Read the model definition and answer for the solid it produces. Units are mm, in the model's axes. Give positions to 0.01 mm unless a question says otherwise; leave off trailing zeros. Order: outer loops, then holes, each group sorted by start corner. A loop starts at its lowest first (then second) coordinate and runs counter-clockwise, first axis right, second up. Notation, with made-up numbers: (23, 8) -> (58, 8) arc R17 ccw to (58, 39) -> close; hole circle Ø2 at (76.25, 24). An arc over 180 degrees is marked (long way). Answer as CSV lines item,"result". Start each with the question number.
1) Find section B-B (z = 2.5). Determine the outline of the cut face in (x, y).
2) Straight lines are drawn through the part: L1, parallel to X at y = 8, z = 3; L2, parallel to Y at x = -11.5, z = 5.5; L3, parallel to Z at x = 9, y = -3.5. For each, find the intervals that lie inside material, in ascending order. Write a range as from..to.
3) Find section A-A (y = 4). Determine the outline of the cut face in (x, z).
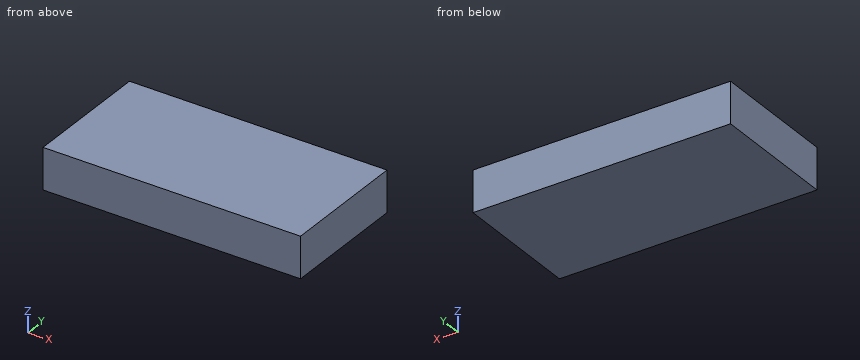
```python
from build123d import *

# Parameters (mm, degrees)
SKETCH_W     = 100
SKETCH_H     = 50
PAD_DEPTH    = 6
SKETCH001_W  = 40
SKETCH001_H  = 20
POCKET_DEPTH = 5
SKETCH003_W  = 100
SKETCH003_H  = 50
PAD001_DEPTH = 10


with BuildPart() as part:
    # Sketch → Pad (new body)
    with BuildSketch(Plane.XY):
        Rectangle(SKETCH_W, SKETCH_H)
    extrude(amount=PAD_DEPTH)

    # Sketch001 (on Face6 of Pad) → Pocket (cut)
    with BuildSketch(Plane.XY.offset(6)):
        Rectangle(SKETCH001_W, SKETCH001_H)
    extrude(amount=-POCKET_DEPTH, mode=Mode.SUBTRACT)

    # Sketch003 (on Face5 of Pocket) → Pad001 (join)
    with BuildSketch(Plane.XY.offset(6)):
        Rectangle(SKETCH003_W, SKETCH003_H)
    extrude(amount=PAD001_DEPTH)


solid = part.part
```
Findings below:
1,outline,"(-50, -25) -> (50, -25) -> (50, 25) -> (-50, 25) -> close; hole (-20, -10) -> (20, -10) -> (20, 10) -> (-20, 10) -> close"
2,L1,"-50..-20, 20..50"
2,L2,"-25..-10, 10..25"
2,L3,"0..1, 6..16"
3,outline,"(-50, 0) -> (50, 0) -> (50, 16) -> (-50, 16) -> close; hole (-20, 1) -> (20, 1) -> (20, 6) -> (-20, 6) -> close"
